Verification items for the finished model (mm, model axes). A direction names the side the tool comes from. Coordinates: 2 decimals unless noted, no trailing zeros. Write each loop counter-clockwise with the first axis right and the second up, starting at its lowest first coordinate (ties: lowest second). Pieces come first, ordered by that corner, then holes. Notation, with made-up numbers: (-0.75, -24) -> (41.25, -24) arc R22 cw to (41.25, -3) -> close; hole circle Ø5 at (72, -26). An arc over 180 degrees is marked (long way). Write each question's results on one line, items separated by ' | '. Start each with the question number.
from build123d import *

# Parameters (mm, degrees)
F0_R            = 55
F1_DEPTH        = 2
F2_R            = 20
F2_R_2          = 18
F3_DEPTH        = 650
F4_R            = 18
F4_R_2          = 16
F5_DEPTH        = 25
F5_DEPTH_BACK   = 25
F6_R            = 22
F7_DEPTH        = 2
F8_R            = 3
F9_DEPTH        = 2.001
F9_COPIES_COUNT = 5


# Not quite as in the source:
# - a pattern or mirror of a feature is missing from the dataset's text; its kind, count and spacing are read off the source's solid


with BuildPart() as f1:
    # F0 (on Top) → F1 (new body)
    with BuildSketch(Plane.XY):
        Circle(F0_R)
    extrude(amount=F1_DEPTH)

    # F2 (on face) → F3 (join)
    with BuildSketch(Plane(origin=(0, 0, 0), x_dir=(1, 0, 0), z_dir=(0, 0, -1))):
        Circle(F2_R)
        Circle(F2_R_2, mode=Mode.SUBTRACT)
    extrude(amount=F3_DEPTH)

    # F4 (on face) → F5 (join, two sides)
    with BuildSketch(Plane(origin=(0, 0, -650), x_dir=(1, 0, 0), z_dir=(0, 0, -1))) as f5_sk:
        Circle(F4_R)
        Circle(F4_R_2, mode=Mode.SUBTRACT)
    extrude(amount=F5_DEPTH)
    extrude(f5_sk.sketch, amount=-F5_DEPTH_BACK)

    # F6 (on face) → F7 (join)
    with BuildSketch(Plane(origin=(0, 0, -675), x_dir=(1, 0, 0), z_dir=(0, 0, -1))):
        Circle(F6_R)
    extrude(amount=F7_DEPTH)

    # F8 (on face) → F9 (cut, through all)
    with BuildSketch(Plane(origin=(0, 0, 0), x_dir=(1, 0, 0), z_dir=(0, 0, -1))):
        with Locations((0, -40)):
            Circle(F8_R)
    f9 = extrude(amount=-F9_DEPTH, mode=Mode.SUBTRACT)

    # F9_copies: F9 ×5 about axis
    f9_copies_axis = Axis((0, 0, 0), (0, 0, 1))
    for i in range(1, F9_COPIES_COUNT):
        add(f9.rotate(f9_copies_axis, i * 360 / F9_COPIES_COUNT), mode=Mode.SUBTRACT)


solid = f1.part
1. Sectioned sample at A-A on y = 0. Record the cut outline in (x, z).
2. Mould release check, pull along X, two halves, no side actions. Record for faces 1 (the cylindrical face through (-4.769, 21.477, -675.986)), 2 (the cylindrical face through (-2.343, -17.847, -308.125)), 3 (the flat face through (0, 0, -677)): +X half, -X half, draft (parallel to the pull), parting line (faces both ways), or undercut.
3. Depth check by flat-ended pin: pin 1 Ø3 at (x, z) = (-12.5, -301.5) entering from +Y; pin 2 Ø10 at (x, z) = (17.5, -477.5) entering from +Y; pin 3 Ø9.5 at (x, y) = (38.04, 12.36) entering from -Z. Enter the tip coordinate at first touch or a pass-through.
4. Sectioned sample at B-B on z = -448. Record the cut outline in (x, y), plus the area to 3 significant figures.
5. Material ranges on probe 1 along Z at (x, y) = (-21.5, 1.5); probe 2 along X at (y, z) = (2, -608.5); probe 3 along Y at (x, z) = (0, -367), recorded low to high. Write a range as from..to.
6. Tool access check on faces 4 (the cylindrical face through (-11.923, -53.692, 0.986)), 5 (the flat face through (0, 0, -675)). Record the directions out of +Z, -Z, +X, -X, +Y, -Y that give a thin tool (end or side, any length) a straight path to the whole face; none if there is none.
Computed values:
1) outline: (-55, 0) -> (-20, 0) -> (-20, -650) -> (-18, -650) -> (-18, -675) -> (-22, -675) -> (-22, -677) -> (22, -677) -> (22, -675) -> (18, -675) -> (18, -650) -> (20, -650) -> (20, 0) -> (55, 0) -> (55, 2) -> (-55, 2) -> close; hole (-18, -625) -> (-16, -625) -> (-16, -675) -> (16, -675) -> (16, -625) -> (18, -625) -> (18, 0) -> (-18, 0) -> close
2) face 1: parting line | face 2: undercut | face 3: draft
3) pin 1: stops at y = 16.7 | pin 2: stops at y = 15.61 | pin 3: stops at z = 0
4) outline: circle Ø40 at (0, 0); hole circle Ø36 at (0, 0) | area: 239 mm^2
5) probe 1: z = -677..-675, 0..2 | probe 2: x = -19.9..-17.89, 17.89..19.9 | probe 3: y = -20..-18, 18..20
6) face 4: +Z, -Z | face 5: none
